Here's how the part is built. I have some questions about the finished solid (model axes, mm). A direction names the side the tool comes from. Give positions to 0.01 mm unless a question says otherwise; leave off trailing zeros. Write each loop counter-clockwise with the first axis right and the second up, starting at its lowest first coordinate (ties: lowest second). Pieces come first, ordered by that corner, then holes. Notation, with made-up numbers: (62.25, 84) -> (116.25, 84) arc R7 cw to (116.25, 94) -> close; hole circle Ø10 at (78, 44). An arc over 180 degrees is marked (long way). Use one line per item in the form item = value.
```python
from build123d import *

# Parameters (mm, degrees)
F0_W      = 160
F0_H      = 160
F1_DEPTH  = 15
F2_R      = 15
F3_DEPTH  = 25
F4_R      = 17.5
F5_DEPTH  = 10
F6_R      = 10
F7_W      = 60
F7_H      = 70
F8_DEPTH  = 10
F9_R      = 19.125
F10_DEPTH = 25
F11_R     = 3.25
F12_DEPTH = 25
F13_R     = 3.25
F14_DEPTH = 25


with BuildPart() as f1:
    # F0 (on Front) → F1 (new body)
    with BuildSketch(Plane.XZ):
        Rectangle(F0_W, F0_H)
    extrude(amount=F1_DEPTH)

    # F2 (on face) → F3 (cut)
    with BuildSketch(Plane.XZ.offset(15)):
        Circle(F2_R)
    extrude(amount=-F3_DEPTH, mode=Mode.SUBTRACT)

    # F4 (on face) → F5 (cut)
    with BuildSketch(Plane.XZ.offset(15)):
        Circle(F4_R)
    extrude(amount=-F5_DEPTH, mode=Mode.SUBTRACT)

    # F6
    f6_edges = [f1.edges().sort_by_distance(p)[0] for p in [
        (80, -7.5, 80),
        (80, -7.5, -80),
        (-80, -7.5, -80),
        (-80, -7.5, 80),
    ]]
    fillet(f6_edges, radius=F6_R)

    # F7 (on face) → F8 (cut)
    with BuildSketch(Plane.XZ.offset(15)):
        with Locations((50, 0)):
            Rectangle(F7_W, F7_H)
    extrude(amount=-F8_DEPTH, mode=Mode.SUBTRACT)

    # F9 (on face) → F10 (cut)
    with BuildSketch(Plane(origin=(0, 0, 0), x_dir=(-1, 0, 0), z_dir=(0, 1, 0))):
        with Locations((-50, 0)):
            Circle(F9_R)
    extrude(amount=-F10_DEPTH, mode=Mode.SUBTRACT)

    # F11 (on face) → F12 (cut)
    with BuildSketch(Plane.XZ.offset(5)):
        with Locations((26.45, 23.55)):
            Circle(F11_R)
        with Locations((26.45, -23.55)):
            Circle(F11_R)
        with Locations((73.55, -23.55)):
            Circle(F11_R)
        with Locations((73.55, 23.55)):
            Circle(F11_R)
    extrude(amount=-F12_DEPTH, mode=Mode.SUBTRACT)

    # F13 (on face) → F14 (cut)
    with BuildSketch(Plane.XZ.offset(15)):
        with Locations((70, 70)):
            Circle(F13_R)
        with Locations((70, -68.258837)):
            Circle(F13_R)
        with Locations((-70, -70)):
            Circle(F13_R)
        with Locations((-70, 70)):
            Circle(F13_R)
    extrude(amount=-F14_DEPTH, mode=Mode.SUBTRACT)


solid = f1.part
```
Q1. If we mould it in two halves opening along X, with no side actions, what happens to faces 4 (the face through (20, -10, 0)), 5 (the face through (-14.985, -2.535, 0.66)), 6 (the face through (-77.15, -7.6, -76.99))? For each: +X half, -X half, draft (parallel to the pull), parting line (faces both ways), or undercut.
Result set:
face_4 = +X half
face_5 = undercut
face_6 = -X half
Q2. If I drill on line 1 along Z through (x, y) = (26.45, -3.5); line 2 along Z through (x, y) = (27, -6); line 3 along Z through (x, y) = (0, -8.75), over which ranges is the centre line in solid material (lowest first)? Write a range as from..to.
Result set:
line_1 = -80..-26.8, -20.3..20.3, 26.8..80
line_2 = -80..-35, 35..80
line_3 = -80..-17.5, 17.5..80
Q3. I want a section at D-D, the plane x = 0. Write out the boundary of the cut face in (y, z), and give its area (3 significant figures).
Result set:
outline = (-15, -80) -> (0, -80) -> (0, -15) -> (-5, -15) -> (-5, -17.5) -> (-15, -17.5) -> close; (-15, 17.5) -> (-5, 17.5) -> (-5, 15) -> (0, 15) -> (0, 80) -> (-15, 80) -> close
area = 1,900 mm2
Q4. I want a section at C-C, the plane y = -10.25. Write out the boundary of the cut face in (x, z).
Result set:
outline = (-80, -70) arc R10 ccw to (-70, -80) -> (70, -80) arc R10 ccw to (80, -70) -> (80, -35) -> (20, -35) -> (20, 35) -> (80, 35) -> (80, 70) arc R10 ccw to (70, 80) -> (-70, 80) arc R10 ccw to (-80, 70) -> close; hole circle Ø6.5 at (-70, -70); hole circle Ø6.5 at (-70, 70); hole circle Ø35 at (0, 0); hole circle Ø6.5 at (70, -68.26); hole circle Ø6.5 at (70, 70)
Q5. Which directions (+Z, -Z, +X, -X, +Y, -Y) give clear straight access to the entire face, cutting with the end or side of a thin tool? Please do faces 1 (the face through (50, -10, -35)), 2 (the face through (-72.579, -7.605, 68.022)), 3 (the face through (13, -5, 8)).
Result set:
face_1 = +X, -Y
face_2 = +Y, -Y
face_3 = -Y
Q6. I want a section at A-A, the plane x = 50. Write out the boundary of the cut face in (y, z) (3 decimals), and give its area (3 significant figures).
Result set:
outline = (-15, -80) -> (0, -80) -> (0, -19.125) -> (-5, -19.125) -> (-5, -35) -> (-15, -35) -> close; (-15, 35) -> (-5, 35) -> (-5, 19.125) -> (0, 19.125) -> (0, 80) -> (-15, 80) -> close
area = 1,510 mm2
Q7. I want a section at B-B, the plane z = -23.55. Write out the boundary of the cut face in (x, y).
Result set:
outline = (-80, -15) -> (20, -15) -> (20, -5) -> (23.2, -5) -> (23.2, 0) -> (-80, 0) -> close; (29.7, -5) -> (70.3, -5) -> (70.3, 0) -> (29.7, 0) -> close; (76.8, -5) -> (80, -5) -> (80, 0) -> (76.8, 0) -> close
